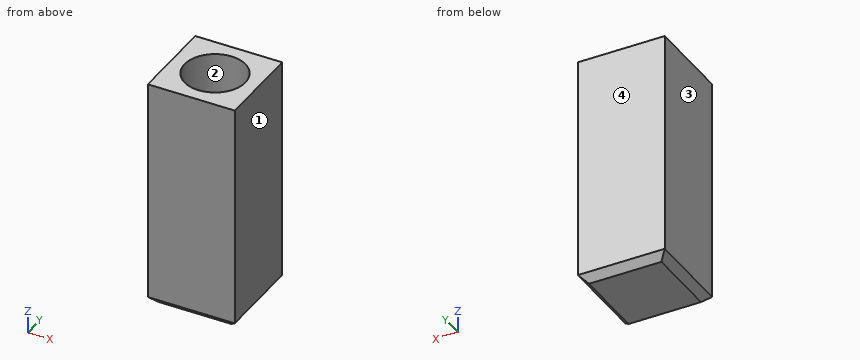
```python
from build123d import *

# Parameters (mm, degrees)
BOSS_EXTRUDE1_DEPTH   = 16
M5_TAPPED_HOLE1_D     = 4.2
M5_TAPPED_HOLE1_DEPTH = 14
M5_TAPPED_HOLE1_TIP   = 1.2618073
CHAMFER1_SIZE         = 0.5


with BuildPart() as part:
    # Sketch1 → Boss-Extrude1 (new body)
    with BuildSketch(Plane.XY):
        with BuildLine():
            Line((-2.998955183, 3), (-2.998955183, 0.079169503))
            ThreePointArc((-2.998955183, 0.079169503), (-2.093142553, 2.14912872), (0, 3))
            Line((0, 3), (-2.998955183, 3))
        make_face()
        with BuildLine():
            ThreePointArc((0, 3), (2.093142553, 2.14912872), (2.998955183, 0.079169503))
            Line((2.998955183, 0.079169503), (2.998955183, 3))
            Line((2.998955183, 3), (0, 3))
        make_face()
        with BuildLine():
            ThreePointArc((-2.998955183, -0.079169503), (-2.093142553, -2.14912872), (0, -3))
            ThreePointArc((0, -3), (2.093142553, -2.14912872), (2.998955183, -0.079169503))
            Line((2.998955183, -0.079169503), (2.998955183, 0.079169503))
            ThreePointArc((2.998955183, 0.079169503), (2.093142553, 2.14912872), (0, 3))
            ThreePointArc((0, 3), (-2.093142553, 2.14912872), (-2.998955183, 0.079169503))
            Line((-2.998955183, 0.079169503), (-2.998955183, -0.079169503))
        make_face()
        with BuildLine():
            ThreePointArc((2.998955183, -0.079169503), (2.093142553, -2.14912872), (0, -3))
            Line((0, -3), (2.998955183, -3))
            Line((2.998955183, -3), (2.998955183, -0.079169503))
        make_face()
        with BuildLine():
            Line((-2.998955183, -0.079169503), (-2.998955183, -3))
            Line((-2.998955183, -3), (0, -3))
            ThreePointArc((0, -3), (-2.093142553, -2.14912872), (-2.998955183, -0.079169503))
        make_face()
    extrude(amount=BOSS_EXTRUDE1_DEPTH)

    # M5 Tapped Hole1
    with Locations(Plane.XY.offset(16)):
        with Locations((0, 0)):
            Hole(M5_TAPPED_HOLE1_D / 2, depth=M5_TAPPED_HOLE1_DEPTH)
            with Locations((0, 0, -(M5_TAPPED_HOLE1_DEPTH + M5_TAPPED_HOLE1_TIP / 2))):  # 118° drill point
                Cone(0, M5_TAPPED_HOLE1_D / 2, M5_TAPPED_HOLE1_TIP, mode=Mode.SUBTRACT)

    # Chamfer1
    chamfer1_edges = [part.edges().sort_by_distance(p)[0] for p in [
        (0, 3, 0),
        (2.998955183, 0, 0),
        (0, -3, 0),
        (-2.998955183, 0, 0),
    ]]
    chamfer(chamfer1_edges, length=CHAMFER1_SIZE)


solid = part.part
```
Work out the finished part from the listing and answer in its coordinate system (mm). Face numbers are marked on the shaded views. Give positions to 0.01 mm unless a question says otherwise; leave off trailing zeros. Order: outer loops, then holes, each group sorted by start corner. A loop starts at its lowest first (then second) coordinate and runs counter-clockwise, first axis right, second up.
1. The mould has two halves that part along X. Classify the marked faces 1, 2, 3 and 4: released by +X, released by -X, zero draft, split by the parting line, or undercut.
Result sheet:
face 1: released by +X
face 2: undercut
face 3: released by -X
face 4: zero draft
2. Section B-B, the plane y = 2.75 is taken. Determine the outline of the cut face in (x, z), and give its area (3 significant figures).
Result sheet:
outline: (-3, 0.5) - (-2.75, 0.25) - (2.75, 0.25) - (3, 0.5) - (3, 16) - (-3, 16) - close
area: 94.4 mm2
3. Straight lines are drawn through the part: L1, parallel to Y at x = 0, z = 8; L2, parallel to Y at x = -1.9, z = 6.25. For each, find the intervals that lie inside material, in ascending order.
Result sheet:
L1: y = -3 to -2.1, 2.1 to 3
L2: y = -3 to -0.89, 0.89 to 3
4. Section A-A, the plane z = 5.75 is taken. Determine the outline of the cut face in (x, y), and give its area (3 significant figures).
Result sheet:
outline: (-3, -3) - (3, -3) - (3, 3) - (-3, 3) - close; hole circle Ø4.2 at (0, 0)
area: 22.1 mm2
